The listing builds one solid part. Answer for the finished solid, in the listing's coordinates (mm). A direction names the side the tool comes from. Coordinates: 2 decimals unless noted, no trailing zeros. Order: outer loops, then holes, each group sorted by start corner. A loop starts at its lowest first (then second) coordinate and runs counter-clockwise, first axis right, second up. Notation, with made-up numbers: (-36, 24) - (22, 24) arc R21 ccw to (22, 47) - close; hole circle Ø2 at (18.25, 35). An arc over 180 degrees is marked (long way). Use a Markdown table: item, result. Add a question column.
Item 1: Find the intervals of material crossed by line 1 along Z through (x, y) = (0, 3.5); line 2 along Z through (x, y) = (0, 8.1); line 3 along X through (y, z) = (9.15, -16), in increasing order.
Item 2: The part is cut by section C-C, the plane y = 8.5. Give the vertices of the cut face in (x, z), then the cut area to 3 significant figures.
Item 3: The part is cut by section A-A, the plane y = 1.5. Give the vertices of the cut face in (x, z).
Item 4: Flat-ended cylindrical pins translate along their axes: P1, Ø3, axis at y = 3, z = -16, coming from the -X side; P2, Ø4, axis at x = 2.5, z = -14.5, coming from the -Y side; P3, Ø1, axis at y = 5.5, z = -21, coming from the +X side. Find the tip coordinate at first contact, or state that the pin passes through.
Item 5: For faces 5 (the flat face through (6.55, 3, -16)), 6 (the flat face through (0, 0, 0)), determine the directions among +Z, -Z, +X, -X, +Y, -Y from which every point of the face is accessible in a straight line to the end or side of a thin tool.
Item 6: The mould has two halves that part along Z. Classify faces 1 (the flat face through (3.321, 2.958, -21.646)), 2 (the flat face through (-6.55, 3, -16)), 3 (the flat face through (0, 10, 0)), 4 (the cylindrical face through (29.97, 1.97, -1.32)): released by +Z, released by -Z, zero draft, split by the parting line, or undercut.
Item 7: The part is cut by section B-B, the plane z = 0. Give the vertices of the cut face in (x, y), then the cut area to 3 significant figures.
Autodesk Inventor part; units mm, degrees
ref_plane "YZ Plane" through (0, 0, 0) normal (1, 0, 0) x (0, 1, 0)
ref_plane "XZ Plane" through (0, 0, 0) normal (0, 1, 0) x (-1, 0, 0)
ref_plane "XY Plane" through (0, 0, 0) normal (0, 0, 1) x (1, 0, 0)
sketch "Sketch1" plane through (0, 0, 0) normal (0, 1, 0) x (-1, 0, 0)
  circle A0 centre (0, 0) radius 30
  circle A1 centre (0, -16) radius 4.25
  dimension "d0" = 60
  dimension "d1" = 8.5
  dimension "d2" = 16
extrude "Extrusion1" add sketch "Sketch1" along normal blind 10
sketch "Sketch2" plane through (0, 0, 0) normal (0, -1, 0) x (1, 0, 0)
  circle A0 centre (0, -16) radius 4.25 construction
  line L0 (6.55, -19.7816) -> (0, -23.5633)
  line L1 (0, -23.5633) -> (-6.55, -19.7816)
  line L2 (-6.55, -19.7816) -> (-6.55, -12.2184)
  line L3 (-6.55, -12.2184) -> (0, -8.4367)
  line L4 (0, -8.4367) -> (6.55, -12.2184)
  line L5 (6.55, -12.2184) -> (6.55, -19.7816)
  point P0 (0, 0)
  dimension "d5" = 13.1
extrude "Extrusion2" cut sketch "Sketch2" against normal blind 6
fillet "Fillet1" radius 6 1 edges at (30, 10, 0)
properties part number "base" material "PC/ABS Plastic"
Solution:
| question | item | result |
|---|---|---|
| 1 | line 1 | z = -30 to -23.56, -8.44 to 30 |
| 1 | line 2 | z = -28.38 to -20.25, -11.75 to 28.38 |
| 1 | line 3 | x = -21.85 to -4.25, 4.25 to 21.85 |
| 2 | outline | circle Ø55.94 at (0, 0); hole circle Ø8.5 at (0, -16) |
| 2 | area | 2,400 mm2 |
| 3 | outline | circle Ø60 at (0, 0); hole (-6.55, -19.78) - (0, -23.56) - (6.55, -19.78) - (6.55, -12.22) - (0, -8.44) - (-6.55, -12.22) - close |
| 4 | P1 | stops at x = -26.26 |
| 4 | P2 | stops at y = 6 |
| 4 | P3 | stops at x = 21.67 |
| 5 | face 5 | -Y |
| 5 | face 6 | +Z, -Z, +X, -X, -Y |
| 6 | face 1 | undercut |
| 6 | face 2 | undercut |
| 6 | face 3 | zero draft |
| 6 | face 4 | split by the parting line |
| 7 | outline | (-30, 0) - (30, 0) - (30, 4) arc R6 ccw to (24, 10) - (-24, 10) arc R6 ccw to (-30, 4) - close |
| 7 | area | 585 mm2 |
